Read the model definition and answer for the solid it produces. Units are mm, in the model's axes. A direction names the side the tool comes from. Coordinates: 2 decimals unless noted, no trailing zeros. Order: outer loops, then holes, each group sorted by start corner. A loop starts at its lowest first (then second) coordinate and runs counter-clockwise, first axis right, second up. Notation, with made-up numbers: (81, -35.75) -> (132, -35.75) arc R26 ccw to (132, 0.25) -> close; hole circle Ø11 at (43, 65). An arc over 180 degrees is marked (long way). Use CSV: the item, a comma, the result in double quotes.
Autodesk Inventor part; units mm, degrees
ref_plane "YZ Plane" through (0, 0, 0) normal (1, 0, 0) x (0, 1, 0)
ref_plane "XZ Plane" through (0, 0, 0) normal (0, 1, 0) x (-1, 0, 0)
ref_plane "XY Plane" through (0, 0, 0) normal (0, 0, 1) x (1, 0, 0)
sketch "Sketch1" plane through (0, 0, 0) normal (1, 0, 0) x (0, 1, 0)
  line L0 (-5.5714, 4.25) -> (5.5714, 4.25)
  line L1 (5.5714, 4.25) -> (5.5714, -4.25)
  line L2 (5.5714, -4.25) -> (-5.5714, -4.25)
  line L3 (-5.5714, -4.25) -> (-5.5714, 4.25)
  line L4 (-5.5714, 0.25) -> (5.5714, 0.25) construction
  circle A0 centre (-3.5714, 2.25) radius 2 construction
  line L5 (-2, -4.25) -> (2, -4.25)
  line L6 (2, -4.25) -> (2, 0.25)
  line L7 (2, 0.25) -> (-2, 0.25)
  line L8 (-2, 0.25) -> (-2, -4.25)
  circle A1 centre (3.5714, 2.25) radius 2 construction
  circle A2 centre (0, 36.35) radius 39 construction
  line L9 (-5.5714, -2.25) -> (5.5714, -2.25) construction
  point P0 (0, 0)
  point P1 (-5.5714, 0)
  point P2 (0, -4.25)
  dimension "d0" = 4
  dimension "d1" = 4.5
  dimension "d2" = 11.1427
  dimension "d15" = 4
  dimension "d34" = 78
  dimension "d35" = 38.6
  dimension "d36" = 4.5
extrude "Extrusion1" add sketch "Sketch1" along normal mid plane 3 contours L0 L1 L2 L6 L7 L8 L3
sketch "Sketch4" plane through (-1.5, -5.5714, -4.25) normal (0, -1, 0) x (1, 0, 0)
  line L0 (0, 8.5) -> (3, 8.5)
  line L1 (0, 0) -> (0, 8.5)
  line L2 (3, 0) -> (0, 0)
  line L3 (3, 8.5) -> (3, 0)
  circle A0 centre (2, 2) radius 0.3962
  point P0 (1.5, 4.25)
  dimension "d16" = 0.7925
  dimension "d24" = 2
  dimension "d25" = 6.5
extrude "Extrusion3" cut sketch "Sketch4" against normal through all contours A0
fillet "Fillet1" radius 1 6 edges at (0, 2, 0.25) (0, -2, 0.25) (0, 2, -4.25) (0, -2, -4.25) (0, 5.5714, -4.25) (0, -5.5714, -4.25)
fillet "Fillet1" radius 2 2 edges at (0, 5.5714, 4.25) (0, -5.5714, 4.25)
sketch "Sketch5" plane through (-1.5, 0, 0) normal (-1, 0, 0) x (0, 0, 1)
  line L0 (-0.75, -2) -> (-3.25, -2)
  line L1 (-4.25, -3) -> (-4.25, -4.5714)
  line L2 (-3.25, -5.5714) -> (2.25, -5.5714)
  line L3 (4.25, -3.5714) -> (4.25, 3.5714)
  line L4 (2.25, 5.5714) -> (-3.25, 5.5714)
  line L5 (-4.25, 4.5714) -> (-4.25, 3)
  line L6 (-3.25, 2) -> (-0.75, 2)
  arc A0 (0.25, 1) -> (-0.75, 2) centre (-0.75, 1) ccw
  line L7 (0.25, 1) -> (0.25, -1)
  arc A1 (-0.75, -2) -> (0.25, -1) centre (-0.75, -1) ccw
  line L8 (-0.75, -2) -> (-3.25, -2)
  line L9 (-0.75, -2) -> (0.25, -2)
  arc A2 (-0.75, -2) -> (0.25, -1) centre (-0.75, -1) ccw
  line L10 (0.25, -2) -> (0.25, -5.5714)
  line L11 (-0.75, 2) -> (0.25, 2)
  line L12 (0.25, 2) -> (0.25, 5.5714)
  line L13 (2.25, 5.5714) -> (-3.25, 5.5714)
  line L14 (0.25, 1) -> (0.25, -1)
  arc A3 (4.25, 3.5714) -> (2.25, 5.5714) centre (2.25, 3.5714) ccw
  arc A4 (2.25, -5.5714) -> (4.25, -3.5714) centre (2.25, -3.5714) ccw
  arc A5 (-3.25, 5.5714) -> (-4.25, 4.5714) centre (-3.25, 4.5714) ccw
  arc A6 (-4.25, 3) -> (-3.25, 2) centre (-3.25, 3) ccw
  arc A7 (-3.25, -2) -> (-4.25, -3) centre (-3.25, -3) ccw
  arc A8 (-4.25, -4.5714) -> (-3.25, -5.5714) centre (-3.25, -4.5714) ccw
  point P0 (0, 0)
  point P1 (4.25, 7)
  point P2 (-4.25, 7)
extrude "Extrusion4" cut sketch "Sketch5" against normal blind 1.5 contours A1 L7 A0 L11 L12 L4 A3 L3 A4 L2 L10 L9
hole "Hole2" at (0, -3.5714, 2.25) at (0, 3.5714, 2.25) direction (1, 0, 0) diameter 2.2 end through all
properties part number "+XPanel_AntennaMount" material "Acetal Resin, Black"
Item 1: Straight lines are drawn through the part: line 1 along Y through (x, z) = (0.45, 2.25); line 2 along Y through (x, z) = (0.8, -1.5); line 3 along Z through (x, y) = (0.5, 4.4). For each, find the intervals that lie inside material, in ascending order.
Return value:
line 1,"y = -5.57 to -4.67, -2.47 to 2.47, 4.67 to 5.57"
line 2,"y = -5.57 to -2, 2 to 5.57"
line 3,"z = -4.25 to -2.65, -1.85 to 1.53, 2.97 to 4.07"
Item 2: Find section B-B, the plane x = 0.5. Give the vertices of the cut face in (y, z).
Return value:
outline,"(-5.57, -3.25) arc R1 ccw to (-4.57, -4.25) -> (-3, -4.25) arc R1 ccw to (-2, -3.25) -> (-2, -2.65) -> (-5.57, -2.65) -> close; (-5.57, -1.85) -> (-2, -1.85) -> (-2, -0.75) arc R1 cw to (-1, 0.25) -> (1, 0.25) arc R1 cw to (2, -0.75) -> (2, -1.85) -> (5.57, -1.85) -> (5.57, 2.25) arc R2 ccw to (3.57, 4.25) -> (-3.57, 4.25) arc R2 ccw to (-5.57, 2.25) -> close; (2, -3.25) arc R1 ccw to (3, -4.25) -> (4.57, -4.25) arc R1 ccw to (5.57, -3.25) -> (5.57, -2.65) -> (2, -2.65) -> close; hole circle Ø2.2 at (-3.57, 2.25); hole circle Ø2.2 at (3.57, 2.25)"
Item 3: Find section A-A, the plane x = -1.3. Give the vertices of the cut face in (y, z).
Return value:
outline,"(-5.57, -3.25) arc R1 ccw to (-4.57, -4.25) -> (-3, -4.25) arc R1 ccw to (-2, -3.25) -> (-2, 0.25) -> (-5.57, 0.25) -> close; (2, -3.25) arc R1 ccw to (3, -4.25) -> (4.57, -4.25) arc R1 ccw to (5.57, -3.25) -> (5.57, 0.25) -> (2, 0.25) -> close"
Item 4: Find section C-C, the plane z = -2.25. Give the vertices of the cut face in (x, y), then the cut area to 3 significant figures.
Return value:
outline,"(-1.5, -5.57) -> (0.1, -5.57) -> (0.1, -2) -> (-1.5, -2) -> close; (-1.5, 2) -> (0.1, 2) -> (0.1, 5.57) -> (-1.5, 5.57) -> close; (0.9, -5.57) -> (1.5, -5.57) -> (1.5, -2) -> (0.9, -2) -> close; (0.9, 2) -> (1.5, 2) -> (1.5, 5.57) -> (0.9, 5.57) -> close"
area,"15.8 mm^2"
Item 5: Each of these flat-tipped pins is pushed along its axis until it touches: P1, Ø1, axis at x = 0.5, z = 3, coming from the +Y side; P2, Ø2.5, axis at y = -1, z = 3, coming from the -X side; P3, Ø2, axis at y = -3.57, z = 2.25, coming from the +X side; P4, Ø0.8, axis at x = 0.5, y = 0, coming from the -Z side. Where does it stop, or does it pass through?
Return value:
P1,"stops at y = 5.56"
P2,"stops at x = 0"
P3,"passes through"
P4,"stops at z = 0.25"
Item 6: A tool of negligible diameter and unlimited length cuts with its end or side. For faces 5 (the cylindrical face through (-0.021, 2.301, -3.965)), 6 (the flat face through (0, 2, -2)), 7 (the flat face through (-1, -4, 0.25)), 8 (the flat face through (0, -5.571, -1)), from which of +Z, -Z, +X, -X, +Y, -Y can it reach the whole face along a straight path? Write none if from no direction.
Return value:
face 5,"-Z, +X, -X"
face 6,"-Z, -X"
face 7,"+Z, -X, +Y, -Y"
face 8,"+Z, -Z, +X, -X, -Y"
Item 7: The mould has two halves that part along Z. Classify faces 1 (the flat face through (0, 5.571, -1)), 2 (the cylindrical face through (0.74, 4.97, 3.68)), 3 (the flat face through (0, -4, -4.25)), 4 (the cylindrical face through (0.76, 4.547, 2.758)): +Z half, -Z half, draft (parallel to the pull), parting line (faces both ways), or undercut.
Return value:
face 1,"draft"
face 2,"+Z half"
face 3,"-Z half"
face 4,"undercut"
Item 8: Find section D-D, the plane z = 2. Give the vertices of the cut face in (x, y).
Return value:
outline,"(0, -5.57) -> (1.5, -5.57) -> (1.5, -4.64) -> (0, -4.64) -> close; (0, -2.5) -> (1.5, -2.5) -> (1.5, 2.5) -> (0, 2.5) -> close; (0, 4.64) -> (1.5, 4.64) -> (1.5, 5.57) -> (0, 5.57) -> close"
